from build123d import *

# Parameters (mm, degrees)
F0_R          = 5
F1_DEPTH      = 50
F2_SIZE       = 5
F5_DEPTH      = 5
F5_DEPTH_BACK = 5
F6_DEPTH      = 5
F8_DEPTH      = 16
F10_DEPTH     = 25


with BuildPart() as f1:
    # F0 (on Top) → F1 (new body)
    with BuildSketch(Plane.XY):
        Circle(F0_R)
    extrude(amount=F1_DEPTH)

    # F2
    f2_edges = [f1.edges().sort_by_distance(p)[0] for p in [
        (-5, 0, 0),
    ]]
    chamfer(f2_edges, length=F2_SIZE)

    # F3 (on face) → F5 (join, two sides)
    with BuildSketch(Plane.XY.offset(50)) as f5_sk:
        Polygon((0, -20), (5.3589838486, -20), (14.6410161514, -14.6410161514), (20, -5.3589838486), (20, 5.3589838486), (14.6410161514, 14.6410161514), (5.3589838486, 20), (-5.3589838486, 20), (-14.6410161514, 14.6410161514), (-20, 5.3589838486), (-20, -5.3589838486), (-14.6410161514, -14.6410161514), (-5.3589838486, -20), align=None)
        with BuildLine():
            ThreePointArc((5, 0), (3.5355339059, -3.5355339059), (0, -5))
            ThreePointArc((0, -5), (-3.5355339059, 3.5355339059), (5, 0))
        make_face(mode=Mode.SUBTRACT)
    extrude(amount=F5_DEPTH)
    extrude(f5_sk.sketch, amount=-F5_DEPTH_BACK)

    # F4 (on face) → F6 (join)
    with BuildSketch(Plane.XY.offset(50)):
        with BuildLine():
            ThreePointArc((5, 0), (-3.5355339059, 3.5355339059), (0, -5))
            ThreePointArc((0, -5), (3.5355339059, -3.5355339059), (5, 0))
        make_face()
    extrude(amount=F6_DEPTH)

    # F7 (on face) → F8 (join)
    with BuildSketch(Plane.XY.offset(55)):
        Polygon((0, 5), (-2.0710678119, 5), (-5, 2.0710678119), (-5, -2.0710678119), (-2.0710678119, -5), (2.0710678119, -5), (5, -2.0710678119), (5, 2.0710678119), (2.0710678119, 5), align=None)
    extrude(amount=F8_DEPTH)

    # F9 (on face) → F10 (cut)
    with BuildSketch(Plane(origin=(3.5355339059, 3.5355339059, 0), x_dir=(-0.7071067812, 0.7071067812, 0), z_dir=(0.7071067812, 0.7071067812, 0))):
        with BuildLine():
            ThreePointArc((0, 68.5), (-1.767766953, 64.232233047), (2.5, 66))
            ThreePointArc((2.5, 66), (1.767766953, 67.767766953), (0, 68.5))
        make_face()
    extrude(amount=-F10_DEPTH, mode=Mode.SUBTRACT)


solid = f1.part
Read the model definition and answer for the solid it produces. Units are mm, in the model's axes. A direction names the side the tool comes from. Give positions to 0.01 mm unless a question says otherwise; leave off trailing zeros. Write each loop counter-clockwise with the first axis right and the second up, starting at its lowest first coordinate (ties: lowest second). Pieces come first, ordered by that corner, then holes. Notation, with made-up numbers: (-30.5, 5) - (-22.5, 5) arc R17 ccw to (-22.5, 22) - close; hole circle Ø9 at (-14.5, 51). An arc over 180 degrees is marked (long way). Use CSV: the item, a comma, the result in double quotes. Start each with the question number.
(1) Find section C-C (z = 49). Give the vertices of the cut face in (x, y).
(2) For faces 1 (the flat face through (-5, 0, 63)), 2 (the flat face through (3.556, 3.515, 59.733)), 3 (the flat face through (5, 0, 63)), 4 (the flat face through (4, -4, 45)), 5 (the flat face through (4, -4, 55)), determine the directions among +Z, -Z, +X, -X, +Y, -Y from which every point of the face is accessible in a straight line to the end or side of a thin tool.
(3) Find section B-B (x = -16.5). Give the vertices of the cut face in (y, z).
(4) Find section A-A (z = 60.5). Give the vertices of the cut face in (x, y).
(5) Consider line 1 along Z through (x, y) = (-7.5, 4); line 2 along X through (y, z) = (1, 67); line 3 along Z through (x, y) = (0, -2). Determine where each line is inside the solid, lowest interval first.
(6) Given P1, Ø4.5, axis at x = -0.5, z = 62, coming from the -Y side; P2, Ø5, axis at y = -10, z = 58, coming from the -X side; P3, Ø4, axis at x = -15.5, z = 52.5, coming from the -Y side; P4, Ø12, axis at x = -9, z = 34, coming from the -Y side, each flat-ended and moving along its own axis, determine where each tip first touches the part or whether it passes through.
(7) Find section D-D (y = -10.5). Give the vertices of the cut face in (x, z).
Findings below:
1,outline,"(-20, -5.36) - (-14.64, -14.64) - (-5.36, -20) - (5.36, -20) - (14.64, -14.64) - (20, -5.36) - (20, 5.36) - (14.64, 14.64) - (5.36, 20) - (-5.36, 20) - (-14.64, 14.64) - (-20, 5.36) - close"
2,face 1,"+Z, -X, +Y, -Y"
2,face 2,"+Z, +X, +Y"
2,face 3,"+Z, +X, +Y, -Y"
2,face 4,"-Z"
2,face 5,"+Z"
3,outline,"(-11.42, 45) - (11.42, 45) - (11.42, 55) - (-11.42, 55) - close"
4,outline,"(-5, -2.07) - (-2.07, -5) - (2.07, -5) - (5, -2.07) - (5, 2.07) - (2.07, 5) - (-2.07, 5) - (-5, 2.07) - close"
5,line 1,"45 to 55"
5,line 2,"-5 to -2.24, 4.24 to 5"
5,line 3,"2 to 63.94, 68.06 to 71"
6,P1,"y = -5"
6,P2,"through"
6,P3,"y = -15.3"
6,P4,"y = -4"
7,outline,"(-17.03, 45) - (17.03, 45) - (17.03, 55) - (-17.03, 55) - close"
